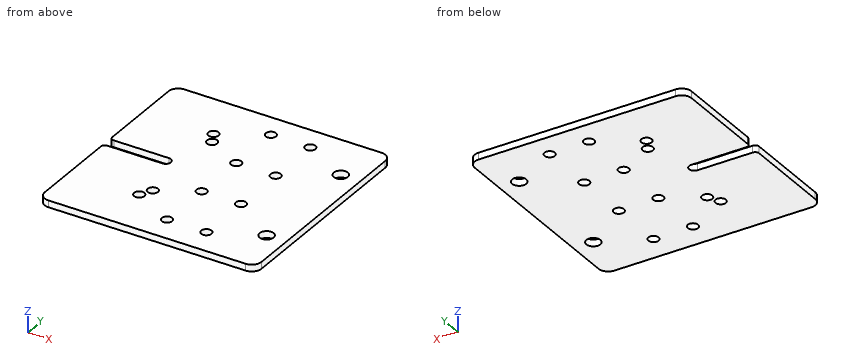
Autodesk Inventor part; units mm, degrees
ref_plane "YZ Plane" through (0, 0, 0) normal (1, 0, 0) x (0, 1, 0)
ref_plane "XZ Plane" through (0, 0, 0) normal (0, 1, 0) x (-1, 0, 0)
ref_plane "XY Plane" through (0, 0, 0) normal (0, 0, 1) x (1, 0, 0)
sketch "Sketch1" plane through (0, 0, 0) normal (0, 0, 1) x (1, 0, 0)
  line L0 (-55, 55) -> (55, 55)
  line L1 (55, 55) -> (55, -55)
  line L2 (55, -55) -> (-55, -55)
  line L3 (-55, -55) -> (-55, 55)
  point P0 (0, 0)
  dimension "d0" = 110
  dimension "d1" = 110
  dimension "d2" = 55
  dimension "d3" = 55
extrude "Extrusion1" add sketch "Sketch1" along normal blind 3.4163
sketch "Sketch2" plane through (0, 0, 3.4163) normal (0, 0, 1) x (1, 0, 0)
  line L0 (55, 55) -> (-55, 55)
  circle A0 centre (45, 30) radius 3.57
  circle A1 centre (45, -30) radius 3.57
  circle A2 centre (-19.6, -30) radius 2.625
  circle A3 centre (-19.6, 30) radius 2.625
  circle A4 centre (-16.5, 24) radius 2.625
  circle A5 centre (-16.5, -24) radius 2.625
  line L1 (-55, -55) -> (55, -55)
  line L2 (55, -55) -> (55, 55)
  point P0 (0, 0)
  dimension "d6" = 7.14
  dimension "d7" = 7.14
  dimension "d8" = 5.25
  dimension "d9" = 5.25
  dimension "d10" = 60
  dimension "d11" = 25
  dimension "d12" = 64.6
  dimension "d13" = 64.6
  dimension "d14" = 60
  dimension "d16" = 25
  dimension "d20" = 5.25
  dimension "d21" = 5.25
  dimension "d22" = 71.5
  dimension "d23" = 31
  dimension "d24" = 31
  dimension "d25" = 71.5
  dimension "d27" = 10
  dimension "d28" = 10
extrude "Extrusion2" cut sketch "Sketch2" against normal through all
sketch "Sketch3" plane through (0, 0, 3.4163) normal (0, 0, 1) x (1, 0, 0)
  line L0 (55, 55) -> (-55, 55)
  arc A0 (-25, -2.625) -> (-25, 2.625) centre (-25, 0) ccw
  line L1 (-55, 55) -> (-55, -55)
  line L2 (-55, 2.625) -> (-25, 2.625)
  line L3 (-25, -2.625) -> (-55, -2.625)
  point P0 (0, 0)
  dimension "d30" = 5.25
  dimension "d33" = 55
  dimension "d38" = 30
  dimension "d39" = 30
extrude "Extrusion3" cut sketch "Sketch3" against normal through all
fillet "Fillet2" radius 5 4 edges at (-55, 55, 1.7082) (-55, -55, 1.7082) (55, 55, 1.7082) (55, -55, 1.7082)
sketch "Sketch4" plane through (0, 0, 3.4163) normal (0, 0, 1) x (1, 0, 0)
  line L0 (50, 55) -> (-50, 55)
  circle A0 centre (1.7, 42.5) radius 2.625
  point P0 (0, 0)
  dimension "d40" = 5.25
  dimension "d50" = 12.5
extrude "Extrusion4" cut sketch "Sketch4" against normal through all
fillet "Fillet3" radius 2 2 edges at (-55, 2.625, 1.7082) (-55, -2.625, 1.7082)
pattern_linear "Rectangular Pattern1" count 2 spacing 20 along (1, 0, 0) count 4 spacing 28 along (0, -1, 0) of "Extrusion4"
equation "\"d13\" = d12"
equation "\"d14\" = d10"
equation "\"d16\" = d11"
equation "\"d24\" = d23"
equation "\"d25\" = d22"
equation "\"d39\" = d38"
properties part number "S2_Zplate" material "Steel, Mild"
Input: part model. Units: mm. Frame: model coordinates. Give positions to 0.01 mm unless a question says otherwise; leave off trailing zeros. Write each loop counter-clockwise with the first axis right and the second up, starting at its lowest first coordinate (ties: lowest second). Pieces come first, ordered by that corner, then holes. Notation, with made-up numbers: (77.25, 28.25) - (108.25, 28.25) arc R12 cw to (108.25, 32.25) - close; hole circle Ø3 at (53.5, 41). An arc over 180 degrees is marked (long way). Write item = value, one per line. Start each with the question number.
1. Section query C-C, the plane z = 1.3. Count the separate pieces of the cut face and the enclosed holes in it, then the cut area to 3 significant figures.
2. Ray query, L1, parallel to Y at x = 21.7, z = 2.6 (3 decimals); L2, parallel to Y at x = -16.5, z = 2.6 (3 decimals); L3, parallel to Y at x = -42, z = 3 (3 decimals). Return the intervals inside material, ascending.
3. Section query B-B, the plane y = 42.5. Output: boundary loops of the cut face in (x, z) (3 decimals), then the cut area to 3 significant figures.
4. Section query D-D, the plane x = -34. Output: boundary loops of the cut face in (y, z) (3 decimals), then the cut area to 3 significant figures.
5. Section query A-A, the plane x = 21.7. Output: boundary loops of the cut face in (y, z) (3 decimals), then the cut area to 3 significant figures.
6. First-contact query: pin 1 Ø4.5 at (x, y) = (21.7, -13.5) entering from +Z. Flat tip, straight axial feed; report the tip coordinate or a pass-through.
Check sheet entries:
q1.separate_pieces = 1
q1.enclosed_holes = 14
q1.area = 11,600 mm2
q2.L1 = -55 to -44.125, -38.875 to -16.125, -10.875 to 11.875, 17.125 to 39.875, 45.125 to 55
q2.L2 = -55 to -26.625, -21.375 to 21.375, 26.625 to 55
q2.L3 = -55 to -2.625, 2.625 to 55
q3.outline = (-55, 0) - (-0.925, 0) - (-0.925, 3.416) - (-55, 3.416) - close; (4.325, 0) - (19.075, 0) - (19.075, 3.416) - (4.325, 3.416) - close; (24.325, 0) - (55, 0) - (55, 3.416) - (24.325, 3.416) - close
q3.area = 340 mm2
q4.outline = (-55, 0) - (-2.625, 0) - (-2.625, 3.416) - (-55, 3.416) - close; (2.625, 0) - (55, 0) - (55, 3.416) - (2.625, 3.416) - close
q4.area = 358 mm2
q5.outline = (-55, 0) - (-44.125, 0) - (-44.125, 3.416) - (-55, 3.416) - close; (-38.875, 0) - (-16.125, 0) - (-16.125, 3.416) - (-38.875, 3.416) - close; (-10.875, 0) - (11.875, 0) - (11.875, 3.416) - (-10.875, 3.416) - close; (17.125, 0) - (39.875, 0) - (39.875, 3.416) - (17.125, 3.416) - close; (45.125, 0) - (55, 0) - (55, 3.416) - (45.125, 3.416) - close
q5.area = 304 mm2
q6.pin_1 = through
